from build123d import *

# Parameters (mm, degrees)
SKETCH1_W                                           = 97.5
SKETCH1_H                                           = 97.5
BOSS_EXTRUDE1_DEPTH                                 = 10
CUT_EXTRUDE4_REACH                                  = 71.664
SKETCH14_R                                          = 12.7
CUT_EXTRUDE5_REACH                                  = 111.466
CUT_EXTRUDE5_END_RADIUS                             = 12.7
SKETCH15_W                                          = 3.175
SKETCH15_H                                          = 10
CUT_EXTRUDE6_REACH                                  = 111.466
CUT_EXTRUDE6_END_RADIUS                             = 12.7
SKETCH16_W                                          = 3.175
SKETCH16_H                                          = 10
CBORE_START                                         = 27.8375
CBORE_FOR_5_BINDING_HEAD_MACHINE_SC_2_R             = 1.7272
CBORE_FOR_5_BINDING_HEAD_MACHINE_SCREW2_DEPTH       = 20.9125
CBORE_START_2                                       = 46.7688
CBORE_FOR_5_BINDING_HEAD_MACHINE_SC_3_O_R           = 3.77063
CBORE_FOR_5_BINDING_HEAD_MACHINE_SC_3_O_R_2         = 1.7272
CBORE_FOR_5_BINDING_HEAD_MACHINE_SC_3_DEPTH         = 1.9812
CBORE_FOR_5_BINDING_HEAD_MACHINE_SCREW3_D           = 3.4544
CBORE_FOR_5_BINDING_HEAD_MACHINE_SCREW3_DEPTH       = 22.0865
CBORE_FOR_5_BINDING_HEAD_MACHINE_SCREW3_CBORE_D     = 7.54126
CBORE_FOR_5_BINDING_HEAD_MACHINE_SCREW3_CBORE_DEPTH = 1.9812
F_1_8_0_125_DIAMETER_HOLE2_D                        = 3.175
CBORE_FOR_8_BINDING_HEAD_MACHINE_SCREW1_D           = 4.4958
CBORE_FOR_8_BINDING_HEAD_MACHINE_SCREW1_CBORE_D     = 9.525
CBORE_FOR_8_BINDING_HEAD_MACHINE_SCREW1_CBORE_DEPTH = 2.667
F_1_4_0_25_DIAMETER_HOLE2_D                         = 6.35


# Read off the part's stored shape, not the designer's step: CBORE for #5 Binding Head Machine Screw2
with BuildPart() as part:
    # Sketch1 → Boss-Extrude1 (new body)
    with BuildSketch(Plane(origin=(0, 0, 0), x_dir=(1, 0, 0), z_dir=(0, 1, 0))):
        Rectangle(SKETCH1_W, SKETCH1_H)
    extrude(amount=BOSS_EXTRUDE1_DEPTH)

    # Sketch14 → Cut-Extrude4 (cut, up to next)
    with BuildSketch(Plane(origin=(0, 10, 0), x_dir=(1, 0, 0), z_dir=(0, 1, 0)), mode=Mode.PRIVATE) as cut_extrude4_sk1:
        with Locations(Location((-23.25, -25.75, 0), (0, 0, 270))):
            Circle(SKETCH14_R)
    cut_extrude4_tool1 = extrude(cut_extrude4_sk1.sketch, amount=-CUT_EXTRUDE4_REACH, mode=Mode.PRIVATE) & part.part
    # Sketch14 → Cut-Extrude4 (cut, up to next)
    with BuildSketch(Plane(origin=(0, 10, 0), x_dir=(1, 0, 0), z_dir=(0, 1, 0)), mode=Mode.PRIVATE) as cut_extrude4_sk2:
        with Locations(Location((27.75, 25.25, 0), (0, 0, 270))):
            Circle(SKETCH14_R)
    cut_extrude4_tool2 = extrude(cut_extrude4_sk2.sketch, amount=-CUT_EXTRUDE4_REACH, mode=Mode.PRIVATE) & part.part
    add(cut_extrude4_tool1.solids().sort_by_distance((-23.25, 10, 25.75))[0], mode=Mode.SUBTRACT)
    add(cut_extrude4_tool2.solids().sort_by_distance((27.75, 10, -25.25))[0], mode=Mode.SUBTRACT)

    # Cut-Extrude5: up to this cylinder (the profile starts outside it)
    cut_extrude5_end = Plane(origin=(-23.25, 5, 25.75), z_dir=(0, 1, 0)) * Cylinder(CUT_EXTRUDE5_END_RADIUS, 249.332, mode=Mode.PRIVATE)
    # Sketch15 → Cut-Extrude5 (cut, up to the surface)
    with BuildSketch(Plane.ZY.offset(48.75), mode=Mode.PRIVATE) as cut_extrude5_sk1:
        with Locations((26.25, 5)):
            Rectangle(SKETCH15_W, SKETCH15_H)
    cut_extrude5_tool1 = extrude(cut_extrude5_sk1.sketch, amount=-CUT_EXTRUDE5_REACH, mode=Mode.PRIVATE) - cut_extrude5_end
    add(cut_extrude5_tool1.solids().sort_by_distance((-48.75, 5, 26.25))[0], mode=Mode.SUBTRACT)

    # Cut-Extrude6: up to this cylinder (the profile starts outside it)
    cut_extrude6_end = Plane(origin=(27.75, 5, -25.25), z_dir=(0, 1, 0)) * Cylinder(CUT_EXTRUDE6_END_RADIUS, 249.332, mode=Mode.PRIVATE)
    # Sketch16 → Cut-Extrude6 (cut, up to the surface)
    with BuildSketch(Plane(origin=(0, 0, -48.75), x_dir=(-1, 0, 0), z_dir=(0, 0, -1)), mode=Mode.PRIVATE) as cut_extrude6_sk1:
        with Locations((-28.25, 5)):
            Rectangle(SKETCH16_W, SKETCH16_H)
    cut_extrude6_tool1 = extrude(cut_extrude6_sk1.sketch, amount=-CUT_EXTRUDE6_REACH, mode=Mode.PRIVATE) - cut_extrude6_end
    add(cut_extrude6_tool1.solids().sort_by_distance((28.25, 5, -48.75))[0], mode=Mode.SUBTRACT)

    # CBORE for _5 Binding Head Machine Sc 2 → CBORE for #5 Binding Head Machine Screw2 (cut)
    with BuildSketch(Plane.XY.offset(CBORE_START)):
        with Locations((-42.4, 5)):
            Circle(CBORE_FOR_5_BINDING_HEAD_MACHINE_SC_2_R)
    extrude(amount=CBORE_FOR_5_BINDING_HEAD_MACHINE_SCREW2_DEPTH, mode=Mode.SUBTRACT)

    # CBORE for _5 Binding Head Machine Sc 3 o → CBORE for _5 Binding Head Machine Sc 3 (cut)
    with BuildSketch(Plane.XY.offset(CBORE_START_2)):
        with Locations((-42.4, 5)):
            Circle(CBORE_FOR_5_BINDING_HEAD_MACHINE_SC_3_O_R)
        with Locations((-42.4, 5)):
            Circle(CBORE_FOR_5_BINDING_HEAD_MACHINE_SC_3_O_R_2, mode=Mode.SUBTRACT)
    extrude(amount=CBORE_FOR_5_BINDING_HEAD_MACHINE_SC_3_DEPTH, mode=Mode.SUBTRACT)

    # CBORE for #5 Binding Head Machine Screw3
    with Locations(Plane(origin=(48.75, 0, 0), x_dir=(0, 0, -1), z_dir=(1, 0, 0))):
        with Locations((42.4, 5)):
            CounterBoreHole(CBORE_FOR_5_BINDING_HEAD_MACHINE_SCREW3_D / 2, CBORE_FOR_5_BINDING_HEAD_MACHINE_SCREW3_CBORE_D / 2, CBORE_FOR_5_BINDING_HEAD_MACHINE_SCREW3_CBORE_DEPTH, depth=CBORE_FOR_5_BINDING_HEAD_MACHINE_SCREW3_DEPTH)

    # 1/8 (0.125) Diameter Hole2 (through all)
    with Locations(Plane(origin=(0, 0, 0), x_dir=(-1, 0, 0), z_dir=(0, -1, 0))):
        with Locations((-13.25, -45.75), (-45.12, -45.75), (-13.25, -17), (-45.12, -17)):
            Hole(F_1_8_0_125_DIAMETER_HOLE2_D / 2)

    # CBORE for #8 Binding Head Machine Screw1 (through all)
    with Locations(Plane(origin=(0, 0, 0), x_dir=(-1, 0, 0), z_dir=(0, -1, 0))):
        with Locations((-31, -40.98776), (-31, -21.01224), (-31, -30.997066185)):
            CounterBoreHole(CBORE_FOR_8_BINDING_HEAD_MACHINE_SCREW1_D / 2, CBORE_FOR_8_BINDING_HEAD_MACHINE_SCREW1_CBORE_D / 2, CBORE_FOR_8_BINDING_HEAD_MACHINE_SCREW1_CBORE_DEPTH)

    # 1/4 (0.25) Diameter Hole2 (through all)
    with Locations(Plane(origin=(0, 0, 0), x_dir=(-1, 0, 0), z_dir=(0, -1, 0))):
        with Locations((-20.87, -32.875), (-41.13, -32.875)):
            Hole(F_1_4_0_25_DIAMETER_HOLE2_D / 2)


solid = part.part
Here's how the part is built. I have some questions about the finished solid (model axes, mm). A direction names the side the tool comes from. Give positions to 0.01 mm unless a question says otherwise; leave off trailing zeros. Order: outer loops, then holes, each group sorted by start corner. A loop starts at its lowest first (then second) coordinate and runs counter-clockwise, first axis right, second up. Notation, with made-up numbers: (65, -5) -> (93, -5) arc R14 cw to (93, 22) -> close; hole circle Ø2 at (-28.75, -15). An arc over 180 degrees is marked (long way). Use a Markdown table: item, result. Add a question column.
Item 1: If we mould it in two halves opening along Z, with no side actions, what happens to faces 5 (the face through (40.442, 5.07, 35.974)), 6 (the face through (-1, 10, -1)), 7 (the face through (39, 5, -48.75))? For each: pulls with the +Z half, pulls with the -Z half, needs draft (parallel to the pull), parting line crosses it, or undercut.
Item 2: Will these pins go through, and if not, where does the flat tip stop? pin 1 (5.5 mm diameter, centred on x = -42.4, y = 5, fed in from +Z); pin 2 (6 mm diameter, centred on x = 31, z = 40.99, fed in from -Y); pin 3 (4 mm diameter, centred on x = 20.87, z = 32.875, fed in from +Y).
Item 3: I need wall thicknesses on line 1 (Z direction, x = -23, y = 4.25); line 2 (Z direction, x = 31, y = 8.75); line 3 (X direction, y = 6.5, z = -39). Which ranges of each line are inside material? Lowest first, please.
Item 4: Imagine slicing it at A-A on x = 13.25. Please give me the cut outline in (y, z), plus the area to 4 significant figures.
Item 5: For faces 1 (the face through (-44, 6, 27.838)), 2 (the face through (30, 2.667, 38.8)), 3 (the face through (46.769, 3, -43)), 4 (the face through (-42, 3, 46.769)), which set-ups out of +Z, -Z, +X, -X, +Y, -Y let a thin tool reach every point of the face, with its end or its side?
Item 6: Imagine slicing it at B-B on z = -26. Please give me the cut outline in (x, y).
Data:
| question | item | result |
|---|---|---|
| 1 | face 5 | undercut |
| 1 | face 6 | needs draft |
| 1 | face 7 | pulls with the -Z half |
| 2 | pin 1 | stops at z = 46.77 |
| 2 | pin 2 | stops at y = 2.67 |
| 2 | pin 3 | passes through |
| 3 | line 1 | z = -48.75 to 13.05, 38.45 to 48.75 |
| 3 | line 2 | z = -48.75 to -37.53, -12.97 to 18.76, 23.26 to 28.75, 33.24 to 38.74, 43.24 to 48.75 |
| 3 | line 3 | x = -48.75 to 26.66, 29.84 to 46.77 |
| 4 | outline | (0, -48.75) -> (10, -48.75) -> (10, 15.41) -> (0, 15.41) -> close; (0, 18.59) -> (10, 18.59) -> (10, 44.16) -> (0, 44.16) -> close; (0, 47.34) -> (10, 47.34) -> (10, 48.75) -> (0, 48.75) -> close |
| 4 | area | 911.5 mm² |
| 5 | face 1 | -X, +Y, -Y |
| 5 | face 2 | -Y |
| 5 | face 3 | +X |
| 5 | face 4 | +Z |
| 6 | outline | (-48.75, 0) -> (15.07, 0) -> (15.07, 10) -> (-48.75, 10) -> close; (40.43, 0) -> (48.75, 0) -> (48.75, 10) -> (40.43, 10) -> close |
